Could you check a few things on this model? Use its own coordinates, in mm. Face numbers are marked on the shaded views. A direction names the side the tool comes from. Give positions to 0.01 mm unless a question says otherwise; leave off trailing zeros. Loops run counter-clockwise (first coordinate to the right, second up) from the corner with the lowest first, then second, coordinate; pieces in that order, holes last. Notation, with made-up numbers: (80, 25.5) -> (130, 25.5) arc R24 ccw to (130, 42.5) -> close; hole circle Ø4 at (83.25, 61). An arc over 180 degrees is marked (long way). Write each question's results on one line, items separated by ' | '. Start each with the question number.
Q1. If we section it at A-A, the plane z = 0: List the corners of the cut face in (x, y) for me, plus the area to 3 significant figures.
Q2. If we section it at D-D, the plane y = 6.75: List the corners of the cut face in (x, z) for me.
Q3. If we section it at B-B, the plane x = 0: List the corners of the cut face in (y, z) for me, plus the area to 3 significant figures.
Q4. We'd pull the mould along X, two halves only. Please class the marked faces 3, 4 and 5: released by +X, released by -X, zero draft, split by the parting line, or undercut.
Q5. Which directions (+Z, -Z, +X, -X, +Y, -Y) give clear straight access to the entire face, cutting with the end or side of a thin tool? Please do the marked faces 1 and 2.
Q6. If we section it at C-C, the plane y = 5: List the corners of the cut face in (x, z) for me, plus the area to 3 significant figures.
Q7. If I drill on line 1 along X through (y, z) = (7.8, 0); line 2 along Y through (x, z) = (1, 1.5); line 3 along Y through (x, z) = (-2, -6.5), over which ranges is the centre line in solid material (lowest first)?
Q8. Will these pins go through, and if not, where does the flat tip stop? P1, Ø2, axis at y = 6, z = 5, coming from the +X side; P2, Ø1, axis at y = 5.5, z = -3, coming from the -X side; P3, Ø1, axis at y = 5.5, z = -3.5, coming from the -X side.
from build123d import *

# Parameters (mm, degrees)
SKETCH1_R           = 7
BOSS_EXTRUDE1_DEPTH = 6.5
SKETCH2_R           = 7
SKETCH2_R_2         = 0.611197666
BOSS_EXTRUDE2_DEPTH = 2
SKETCH3_R           = 2.310970428


with BuildPart() as part:
    # Sketch1 → Boss-Extrude1 (new body)
    with BuildSketch(Plane(origin=(0, 0, 0), x_dir=(1, 0, 0), z_dir=(0, 1, 0))):
        with Locations(Location((0, 0, 0), (0, 0, 270))):  # turned: the seam where the file's is
            Circle(SKETCH1_R)
        with BuildLine():
            Line((-1.88, 1.937937047), (-1.88, -1.937937047))
            ThreePointArc((-1.88, -1.937937047), (0, -2.7), (1.88, -1.937937047))
            Line((1.88, -1.937937047), (1.88, 1.937937047))
            ThreePointArc((1.88, 1.937937047), (0, 2.7), (-1.88, 1.937937047))
        make_face(mode=Mode.SUBTRACT)
    extrude(amount=BOSS_EXTRUDE1_DEPTH)

    # Sketch2 → Boss-Extrude2 (add)
    with BuildSketch(Plane(origin=(0, 6.5, 0), x_dir=(1, 0, 0), z_dir=(0, 1, 0))):
        with Locations(Location((0, 0, 0), (0, 0, 270))):  # turned: the seam where the file's is
            Circle(SKETCH2_R)
        with Locations(Location((0, 0, 0), (0, 0, 270))):  # turned: the seam where the file's is
            Circle(SKETCH2_R_2, mode=Mode.SUBTRACT)
    extrude(amount=BOSS_EXTRUDE2_DEPTH)

    # Sketch3 → Cut-Revolve1 (revolve, cut)
    with BuildSketch(Plane(origin=(0, 0, 0), x_dir=(0, 0, -1), z_dir=(1, 0, 0))):
        with Locations((-7, 4.25)):
            Circle(SKETCH3_R)
    revolve(axis=Axis((0, 0, 0), (0, 1, 0)), mode=Mode.SUBTRACT)


solid = part.part
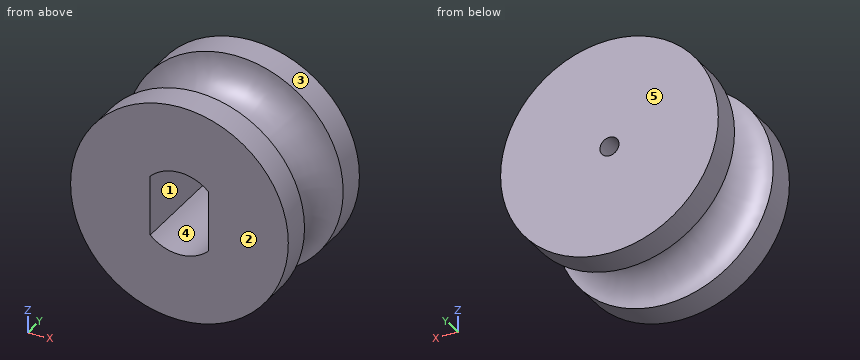
Final values:
1) outline: (-7, 0) -> (-1.88, 0) -> (-1.88, 6.5) -> (-0.61, 6.5) -> (-0.61, 8.5) -> (-7, 8.5) -> (-7, 6.56) arc R2.31 cw to (-7, 1.94) -> close; (0.61, 6.5) -> (1.88, 6.5) -> (1.88, 0) -> (7, 0) -> (7, 1.94) arc R2.31 cw to (7, 6.56) -> (7, 8.5) -> (0.61, 8.5) -> close | area: 75.3 mm²
2) outline: circle Ø14 at (0, 0); hole circle Ø1.22 at (0, 0)
3) outline: (0, -7) -> (1.94, -7) arc R2.31 cw to (6.56, -7) -> (8.5, -7) -> (8.5, -0.61) -> (6.5, -0.61) -> (6.5, -2.7) -> (0, -2.7) -> close; (0, 2.7) -> (6.5, 2.7) -> (6.5, 0.61) -> (8.5, 0.61) -> (8.5, 7) -> (6.56, 7) arc R2.31 cw to (1.94, 7) -> (0, 7) -> close | area: 64.7 mm²
4) face 3: split by the parting line | face 4: undercut | face 5: zero draft
5) face 1: -Y | face 2: +Z, -Z, +X, -X, -Y
6) outline: circle Ø9.63 at (0, 0); hole (-1.88, -1.94) arc R2.7 ccw to (1.88, -1.94) -> (1.88, 1.94) arc R2.7 ccw to (-1.88, 1.94) -> close | area: 54.3 mm²
7) line 1: x = -7 to -0.61, 0.61 to 7 | line 2: y = 6.5 to 8.5 | line 3: y = 0 to 1.95, 6.55 to 8.5
8) P1: stops at x = 5.62 | P2: stops at x = -4.67 | P3: stops at x = -4.33
